Model file for the job. Use its own axes, mm. A direction names the side the tool comes from. Give positions to 0.01 mm unless a question says otherwise; leave off trailing zeros. Write each loop counter-clockwise with the first axis right and the second up, starting at its lowest first coordinate (ties: lowest second). Pieces come first, ordered by that corner, then holes. Notation, with made-up numbers: (-34, 18.25) - (4, 18.25) arc R13 ccw to (4, 32.25) - close; hole circle Ø10 at (-13, 25). An arc over 180 degrees is marked (long way). One line per item, written item: value. Start each with the question number.
(1) Drop flat-ended pins along their axis: P1, Ø1.5, axis at x = 7.5, y = 1.5, coming from the -Z side; P2, Ø10, axis at x = 11, z = -11.5, coming from the -Y side; P3, Ø3.5, axis at x = 6, y = 1, coming from the +Z side; P4, Ø2, axis at x = -13.21, z = 8.03, coming from the +Y side. Give the stop position or say it passes through.
(2) Mould opens along Y. For faces 1 (the face through (0, 0, 0)), 2 (the face through (75, 210, -150)), 3 (the face through (13, 22.138, -3)) say: pulls with the +Y half, pulls with the -Y half, needs draft (parallel to the pull), parting line crosses it, or undercut.
(3) Cut at A-A, the plane z = 18. List the corners of the cut face in (x, y).
(4) Probe L1, parallel to Y at x = 70.5, z = 55; L2, parallel to Z at x = 47.5, y = 132; L3, parallel to Y at x = 71, z = 47.5. List the from-to ranges inside material, lowest first.
(5) 3-axis set-ups, long thin cutter, end or side, ignore diameter. For faces 4 (the face through (75, 210, 150)), 5 (the face through (4, 3, -9)): which of +Z, -Z, +X, -X, +Y, -Y reach the whole face in a straight line?
from build123d import *

# Parameters (mm, degrees)
IZIM1_W                     = 35
IZIM1_H                     = 25
Y_KSEKLIK_EKSTR_ZYON1_DEPTH = 3
IZIM2_R                     = 9
IZIM2_R_2                   = 6.5
IZIM9_R                     = 6.5
IZIM13_R                    = 6.5
Y_KSEKLIK_EKSTR_ZYON3_DEPTH = 150
M3_BO_LUKLU_DELIK1_D        = 3.4
M3_BO_LUKLU_DELIK1_DEPTH    = 3


with BuildPart() as part:
    # Çizim1 → Yükseklik-Ekstrüzyon1 (new body)
    with BuildSketch(Plane(origin=(0, 0, 0), x_dir=(1, 0, 0), z_dir=(0, 1, 0))):
        Rectangle(IZIM1_W, IZIM1_H)
    extrude(amount=Y_KSEKLIK_EKSTR_ZYON1_DEPTH)

    # Süpür1: sweep along a path in Çizim5
    with BuildLine(Plane.XY) as s_p_r1_path:
        Line((0, 3), (7.004599808, 22.138442505))
    # Çizim2 → Süpür1 (sweep)
    with BuildSketch(Plane(origin=(0, 3, 0), x_dir=(1, 0, 0), z_dir=(0, 1, 0))):
        Circle(IZIM2_R)
        Circle(IZIM2_R_2, mode=Mode.SUBTRACT)
    sweep(path=s_p_r1_path.line)

    # Süpür2: sweep along a path in Çizim11
    with BuildLine(Plane.XY) as s_p_r2_path:
        Line((0, 3), (74.882319817, 209.863815538))
    # Çizim9 → Süpür2 (sweep)
    with BuildSketch(Plane(origin=(0, 3, 0), x_dir=(1, 0, 0), z_dir=(0, 1, 0))):
        Circle(IZIM9_R)
    sweep(path=s_p_r2_path.line)

    # Çizim13 → Yükseklik-Ekstrüzyon3 (add, symmetric)
    with BuildSketch(Plane.XY):
        with Locations((74.882319817, 209.863815538)):
            Circle(IZIM13_R)
    extrude(amount=Y_KSEKLIK_EKSTR_ZYON3_DEPTH, both=True)

    # M3 Boşluklu Delik1
    with Locations(Plane(origin=(0, 3, 0), x_dir=(1, 0, 0), z_dir=(0, 1, 0))):
        with Locations((-13.209013164, -8.030166901), (-13.209013164, 9.355779361), (13.345161769, -8.030166901), (13.345161769, 9.355779361)):
            Hole(M3_BO_LUKLU_DELIK1_D / 2, depth=M3_BO_LUKLU_DELIK1_DEPTH)


solid = part.part
Answers follow:
1. P1: stops at z = -12.5
1. P2: stops at y = 0
1. P3: stops at z = 12.5
1. P4: passes through
2. face 1: pulls with the -Y half
2. face 2: needs draft
2. face 3: undercut
3. outline: circle Ø13 at (74.88, 209.86)
4. L1: y = 205.06 to 214.66
4. L2: z = -6.45 to 6.45
4. L3: y = 204.65 to 215.08
5. face 4: +Z, +X, -X, +Y, -Y
5. face 5: none
